Part print with two shaded views. Sizes in mm from the minimum x, y, z corner. A direction names the side the tool comes from. Coordinates: 2 decimals unless noted, no trailing zeros. Order: outer loops, then holes, each group sorted by start corner. A loop starts at its lowest first (then second) coordinate and runs counter-clockwise, first axis right, second up. Notation, with made-up numbers: (-24, 22.5) - (23, 22.5) arc R25 cw to (23, 39.5) - close; hole circle Ø5 at (39, 65.25). An arc over 180 degrees is marked (long way). Return JSON: item names as keys, results as strings.
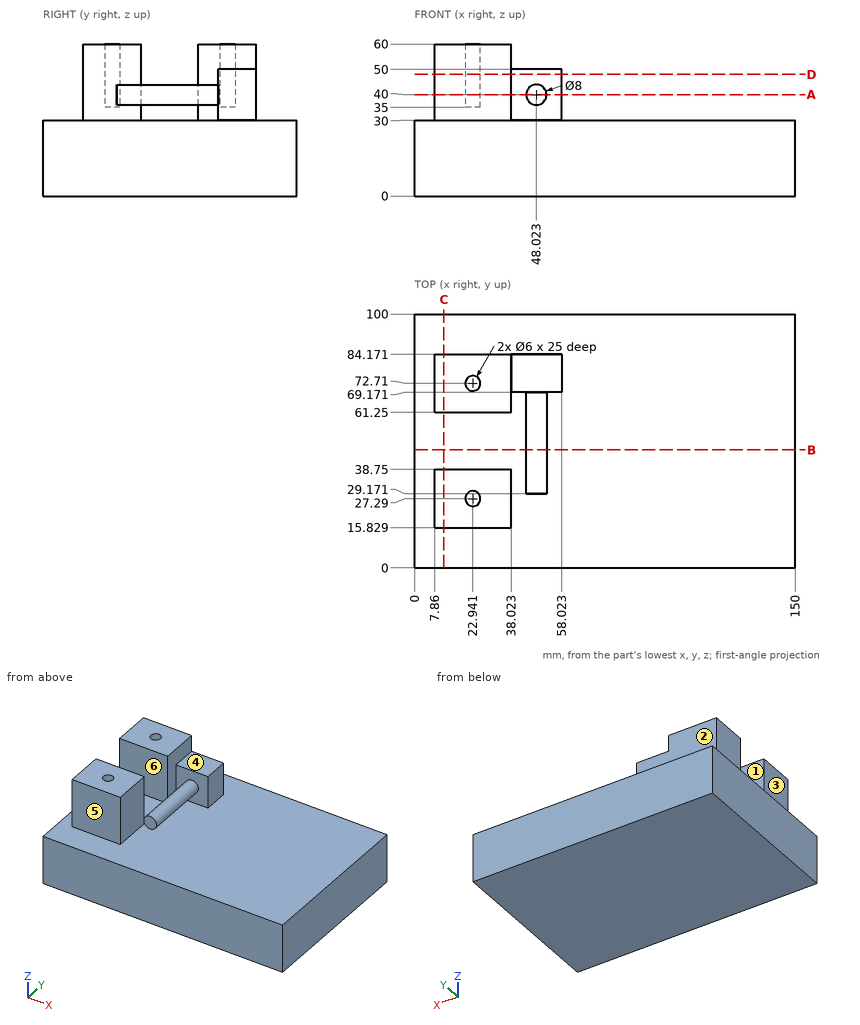
Item 1: Band-saw the part on D-D, the plane z = 48. List the corners of the cut face in (x, y), then the cut area to 3 significant figures.
Findings below:
{"outline": "(7.86, 15.83) - (38.02, 15.83) - (38.02, 38.75) - (7.86, 38.75) - close; (7.86, 61.25) - (38.02, 61.25) - (38.02, 69.17) - (58.02, 69.17) - (58.02, 84.17) - (7.86, 84.17) - close; hole circle Ø6 at (22.94, 27.29); hole circle Ø6 at (22.94, 72.71)", "area": "1,630 mm²"}
Item 2: Mould opens along Y. For the marked faces 1, 2 and 3 say: released by +Y, released by -Y, zero draft, split by the parting line, or undercut.
Findings below:
{"face 1": "undercut", "face 2": "released by +Y", "face 3": "zero draft"}
Item 3: Drop flat-ended pins along their axis: P1, Ø6, axis at x = 51.5, z = 45, coming from the -Y side; P2, Ø6, axis at x = 56.5, z = 44, coming from the -Y side; P3, Ø7.5, axis at x = 44.5, y = 74, coming from the +Z side. Give the stop position or say it passes through.
Findings below:
{"P1": "stops at y = 29.17", "P2": "stops at y = 69.17", "P3": "stops at z = 50"}
Item 4: Band-saw the part on C-C, the plane x = 11.5. List the corners of the cut face in (y, z).
Findings below:
{"outline": "(0, 0) - (100, 0) - (100, 30) - (84.17, 30) - (84.17, 60) - (61.25, 60) - (61.25, 30) - (38.75, 30) - (38.75, 60) - (15.83, 60) - (15.83, 30) - (0, 30) - close"}
Item 5: Band-saw the part on A-A, the plane z = 40. List the corners of the cut face in (x, y), then the cut area to 3 significant figures.
Findings below:
{"outline": "(7.86, 15.83) - (38.02, 15.83) - (38.02, 38.75) - (7.86, 38.75) - close; (7.86, 61.25) - (38.02, 61.25) - (38.02, 69.17) - (44.02, 69.17) - (44.02, 29.17) - (52.02, 29.17) - (52.02, 69.17) - (58.02, 69.17) - (58.02, 84.17) - (7.86, 84.17) - close; hole circle Ø6 at (22.94, 27.29); hole circle Ø6 at (22.94, 72.71)", "area": "1,950 mm²"}
Item 6: Wall check: L1, parallel to X at y = 53, z = 39.5 (1 decimal); L2, parallel to Y at x = 52.5, z = 44; L3, parallel to Y at x = 23, z = 32. Give the ranges that are in metal, low to high. Write a range as [from, to].
Findings below:
{"L1": "x = [44.1, 52]", "L2": "y = [69.17, 84.17]", "L3": "y = [15.83, 38.75], [61.25, 84.17]"}
Item 7: Band-saw the part on B-B, the plane y = 46.5. List the corners of the cut face in (x, z), then the cut area to 3 significant figures.
Findings below:
{"outline": "(0, 0) - (150, 0) - (150, 30) - (0, 30) - close; circle Ø8 at (48.02, 40)", "area": "4,550 mm²"}
Item 8: Which spindle directions (+Z, -Z, +X, -X, +Y, -Y) get a long thin tool onto all of the face, cutting with end or side? Do the marked faces 4, 5 and 6. Say none if no direction does.
Findings below:
{"face 4": "+Z, +X, +Y, -Y", "face 5": "+Z, +X, -X, -Y", "face 6": "+Z, -X"}
